Work out the finished part from the listing and answer in its coordinate system (mm). A direction names the side the tool comes from. Round coordinates to 2 decimals unless told otherwise and drop trailing zeros. Order: outer loops, then holes, each group sorted by start corner. A loop starts at its lowest first (then second) coordinate and runs counter-clockwise, first axis right, second up. Notation, with made-up numbers: (12, 73.5) -> (67, 73.5) arc R5 ccw to (67, 78.5) -> close; hole circle Ø4 at (82, 59.5). An arc over 180 degrees is marked (long way). Use a Markdown table: item, result. Add a question column.
Item 1: A cutting plane is placed at B-B, the plane x = -4. Determine the outline of the cut face in (y, z), plus the area to 3 significant figures.
Item 2: Find the intervals of material crossed by L1, parallel to X at y = -9, z = 0 (3 decimals); L2, parallel to X at y = 26, z = 9; L3, parallel to Y at x = 10, z = -9.5, in increasing order. Write a range as [from, to].
Item 3: For a pull along X with two mould halves and no side action, classify faces 4 (the flat face through (3.526, 11, 8)), 5 (the flat face through (8, 37.727, 0)), 6 (the cylindrical face through (-2.281, 10.142, -11.847)) as +X half, -X half, draft (parallel to the pull), parting line (faces both ways), or undercut.
Item 4: A cutting plane is placed at C-C, the plane x = 10. Determine the outline of the cut face in (y, z).
Item 5: A cutting plane is placed at D-D, the plane z = 13. Determine the outline of the cut face in (x, y), plus the area to 3 significant figures.
Item 6: Flat-ended cylindrical pins translate along their axes: P1, Ø6, axis at x = 0.5, y = 29.5, coming from the +Z side (3 decimals); P2, Ø9.5, axis at y = 0.5, z = 14.5, coming from the +X side; P3, Ø1.5, axis at x = 7, y = 19.5, coming from the -Z side. Find the tip coordinate at first contact, or state that the pin passes through.
Item 7: A cutting plane is placed at A-A, the plane z = 0. Determine the outline of the cut face in (x, y) (3 decimals).
Item 8: A tool of negligible diameter and unlimited length cuts with its end or side. For faces 1 (the flat face through (0, 11, 8)), 2 (the cylindrical face through (-1.598, 11.43, -6.146)), 3 (the flat face through (-4, 35.187, -12)), from which of +Z, -Z, +X, -X, +Y, -Y can it reach the whole face along a straight path? Write none if from no direction.
from build123d import *

# Parameters (mm, degrees)
F2_R     = 6.35
F3_DEPTH = 101.6
F5_DEPTH = 127


with BuildPart() as f1:
    # F0 (on Top) → F1 (revolve)
    with BuildSketch(Plane.XY):
        Polygon((0, 37.726658), (0, -15.613342), (12.065, -15.613342), (12.065, 35.186658), (18.415, 35.186658), (18.415, 37.726658), align=None)
    revolve(axis=Axis((0, 11.056658, 0), (0, -1, 0)))

    # F2 (on face) → F3 (cut)
    with BuildSketch(Plane(origin=(0, 37.726658, 0), x_dir=(-1, 0, 0), z_dir=(0, 1, 0))):
        Circle(F2_R)
    extrude(amount=-F3_DEPTH, mode=Mode.SUBTRACT)

    # F4 (on face) → F5 (cut)
    with BuildSketch(Plane(origin=(0, 37.726658, 0), x_dir=(-1, 0, 0), z_dir=(0, 1, 0))):
        with BuildLine():
            Line((0, 6.35), (0, 18.415))
            ThreePointArc((0, 18.415), (-1.770995, 18.329643), (-3.525572, 18.074362))
            Line((-3.525572, 18.074362), (-3.525572, 5.281367))
            ThreePointArc((-3.525572, 5.281367), (-1.841985, 6.076972), (0, 6.35))
        make_face()
    extrude(amount=-F5_DEPTH, mode=Mode.SUBTRACT)


solid = f1.part
Reported:
| question | item | result |
|---|---|---|
| 1 | outline | (-15.61, -11.38) -> (35.19, -11.38) -> (35.19, -17.98) -> (37.73, -17.98) -> (37.73, -4.93) -> (-15.61, -4.93) -> close; (-15.61, 4.93) -> (37.73, 4.93) -> (37.73, 17.98) -> (35.19, 17.98) -> (35.19, 11.38) -> (-15.61, 11.38) -> close |
| 1 | area | 722 mm² |
| 2 | L1 | [-12.065, -6.35], [6.35, 12.065] |
| 2 | L2 | [-8.04, 0], [3.53, 8.04] |
| 2 | L3 | [35.19, 37.73] |
| 3 | face 4 | undercut |
| 3 | face 5 | draft |
| 3 | face 6 | parting line |
| 4 | outline | (-15.61, -6.75) -> (35.19, -6.75) -> (35.19, -15.46) -> (37.73, -15.46) -> (37.73, 15.46) -> (35.19, 15.46) -> (35.19, 6.75) -> (-15.61, 6.75) -> close |
| 5 | outline | (-13.04, 35.19) -> (0, 35.19) -> (0, 37.73) -> (-13.04, 37.73) -> close; (3.53, 35.19) -> (13.04, 35.19) -> (13.04, 37.73) -> (3.53, 37.73) -> close |
| 5 | area | 57.3 mm² |
| 6 | P1 | z = 12.065 |
| 6 | P2 | x = 7.11 |
| 6 | P3 | z = -10.32 |
| 7 | outline | (-18.415, 35.187) -> (-12.065, 35.187) -> (-12.065, -15.613) -> (-6.35, -15.613) -> (-6.35, 37.727) -> (-18.415, 37.727) -> close; (6.35, -15.613) -> (12.065, -15.613) -> (12.065, 35.187) -> (18.415, 35.187) -> (18.415, 37.727) -> (6.35, 37.727) -> close |
| 8 | face 1 | +Z, +Y, -Y |
| 8 | face 2 | +Y, -Y |
| 8 | face 3 | -Y |
